```python
from build123d import *

# Parameters (mm, degrees)
SKETCH1_W           = 76.2
SKETCH1_H           = 50.8
BOSS_EXTRUDE1_DEPTH = 76.2
SKETCH2_W           = 63.5
SKETCH2_H           = 38.1
CUT_EXTRUDE1_DEPTH  = 71.12
SKETCH3_R           = 3.175
SKETCH3_R_2         = 1.651
CUT_EXTRUDE2_DEPTH  = 48.26
SKETCH4_R           = 1.0922
CUT_EXTRUDE3_DEPTH  = 15.875


with BuildPart() as part:
    # Sketch1 → Boss-Extrude1 (new body)
    with BuildSketch(Plane.XY):
        Rectangle(SKETCH1_W, SKETCH1_H)
    extrude(amount=BOSS_EXTRUDE1_DEPTH)

    # Sketch2 → Cut-Extrude1 (cut)
    with BuildSketch(Plane.XY.offset(76.2)):
        Rectangle(SKETCH2_W, SKETCH2_H)
    extrude(amount=-CUT_EXTRUDE1_DEPTH, mode=Mode.SUBTRACT)

    # Sketch3 → Cut-Extrude2 (cut)
    with BuildSketch(Plane.XY.offset(5.08)):
        Circle(SKETCH3_R)
        with Locations((-16.51, 0)):
            Circle(SKETCH3_R_2)
    extrude(amount=-CUT_EXTRUDE2_DEPTH, mode=Mode.SUBTRACT)

    # Sketch4 → Cut-Extrude3 (cut)
    with BuildSketch(Plane.XY.offset(76.2)):
        with Locations((-35.149835373, 0)):
            Circle(SKETCH4_R)
        with Locations(Location((35.149835373, 0, 0), (0, 0, 180))):
            Circle(SKETCH4_R)
        with Locations((0, 22.186517988)):
            Circle(SKETCH4_R)
        with Locations(Location((0, -22.186517988, 0), (0, 0, 180))):
            Circle(SKETCH4_R)
    extrude(amount=-CUT_EXTRUDE3_DEPTH, mode=Mode.SUBTRACT)


solid = part.part
```
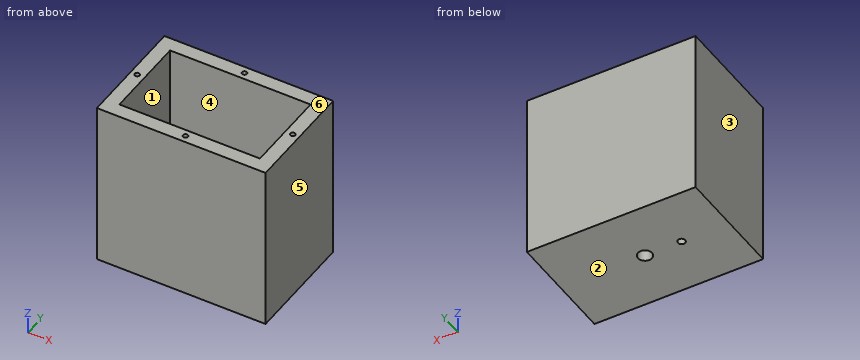
The listing builds one solid part. Answer for the finished solid, in the listing's coordinates (mm). Face numbers are marked on the shaded views. A direction names the side the tool comes from. Give positions to 0.01 mm unless a question says otherwise; leave off trailing zeros. Loops run counter-clockwise (first coordinate to the right, second up) from the corner with the lowest first, then second, coordinate; pieces in that order, holes last. Notation, with made-up numbers: M 19,20.5 L 37,20.5 A14 ccw 37,38.5 Z; hole C 67,69.25 d6. An arc over 180 degrees is marked long. One line per item, written item: value.
Q1. Flat-ended cylindrical pins translate along their axes: P1, Ø11.5, axis at x = 3.5, y = 4, coming from the +Z side; P2, Ø5.5, axis at x = 0, y = 0, coming from the -Z side; P3, Ø1.7, axis at x = -35, y = 0, coming from the +Z side (3 decimals). Find the tip coordinate at first contact, or state that the pin passes through.
Working result:
P1: stops at z = 5.08
P2: passes through
P3: stops at z = 60.325
Q2. Find the intervals of material crossed by line 1 (Y direction, x = 0, z = 65); line 2 (X direction, y = -17, z = 35.5); line 3 (Y direction, x = -24.5, z = 8), in increasing order. Write a range as from..to.
Working result:
line 1: y = -25.4..-23.28, -21.09..-19.05, 19.05..21.09, 23.28..25.4
line 2: x = -38.1..-31.75, 31.75..38.1
line 3: y = -25.4..-19.05, 19.05..25.4
Q3. A cutting plane is placed at B-B on y = 0. Determine the outline of the cut face in (x, z) (3 decimals).
Working result:
outline: M -38.1,0 L -18.161,0 L -18.161,5.08 L -31.75,5.08 L -31.75,76.2 L -34.058,76.2 L -34.058,60.325 L -36.242,60.325 L -36.242,76.2 L -38.1,76.2 Z; M -14.859,0 L -3.175,0 L -3.175,5.08 L -14.859,5.08 Z; M 3.175,0 L 38.1,0 L 38.1,76.2 L 36.242,76.2 L 36.242,60.325 L 34.058,60.325 L 34.058,76.2 L 31.75,76.2 L 31.75,5.08 L 3.175,5.08 Z
Q4. A cutting plane is placed at C-C on x = 29. Determine the outline of the cut face in (y, z), then the cut area to 3 significant figures.
Working result:
outline: M -25.4,0 L 25.4,0 L 25.4,76.2 L 19.05,76.2 L 19.05,5.08 L -19.05,5.08 L -19.05,76.2 L -25.4,76.2 Z
area: 1,160 mm^2
Q5. Determine the mould class of the marked faces 3, 4, 5 and 6 for opening direction X: +X half, -X half, draft (parallel to the pull), parting line (faces both ways), or undercut.
Working result:
face 3: -X half
face 4: undercut
face 5: +X half
face 6: draft
Q6. A cutting plane is placed at D-D on z = 40. Determine the outline of the cut face in (x, y).
Working result:
outline: M -38.1,-25.4 L 38.1,-25.4 L 38.1,25.4 L -38.1,25.4 Z; hole M -31.75,-19.05 L 31.75,-19.05 L 31.75,19.05 L -31.75,19.05 Z
Q7. A cutting plane is placed at A-A on x = 0. Determine the outline of the cut face in (y, z) (3 decimals), then the cut area to 3 significant figures.
Working result:
outline: M -25.4,0 L -3.175,0 L -3.175,5.08 L -19.05,5.08 L -19.05,76.2 L -21.094,76.2 L -21.094,60.325 L -23.279,60.325 L -23.279,76.2 L -25.4,76.2 Z; M 3.175,0 L 25.4,0 L 25.4,76.2 L 23.279,76.2 L 23.279,60.325 L 21.094,60.325 L 21.094,76.2 L 19.05,76.2 L 19.05,5.08 L 3.175,5.08 Z
area: 1,060 mm^2
Q8. For the marked faces 1 and 2, determine the directions among +Z, -Z, +X, -X, +Y, -Y from which every point of the face is accessible in a straight line to the end or side of a thin tool.
Working result:
face 1: +Z
face 2: -Z, +X, -X, +Y, -Y
